Could you check a few things on this drawing? It's one solid part, dimensions in mm from its lowest x, y, z. Round coordinates to 2 decimals unless told otherwise and drop trailing zeros. Write each loop counter-clockwise with the first axis right and the second up, starting at its lowest first coordinate (ties: lowest second). Pieces come first, ordered by that corner, then holes. Notation, with made-up numbers: (20.25, 39) - (51.25, 39) arc R22 cw to (51.25, 72) - close; hole circle Ø9 at (24, -4.5). An arc over 180 degrees is marked (long way). One line per question, with ' | ' between items. Start each with the question number.
(1) Imagine slicing it at B-B (z = 4.25). Write out the boundary of the cut face in (x, y).
(2) Imagine slicing it at C-C (y = 0.5). Write out the boundary of the cut face in (x, z).
(3) Thinking about a two-plate mould opening in Z: for the marked faces 1, 2 and 3, which applies, pulls with the +Z half, pulls with the -Z half, needs draft (parallel to the pull), parting line crosses it, or undercut?
(4) If I drill on L1, parallel to X at y = 0.35, z = 3.65; L2, parallel to X at y = 0.7, z = 2.5; L3, parallel to Z at x = 1.25, y = 0.6, over which ranges is the centre line in solid material (lowest first)?
(5) Imagine slicing it at D-D (x = 0.7). Write out the boundary of the cut face in (y, z).
(6) Will this pin go through, and if not, where does the flat tip stop? pin 1 (1.6 mm diameter, centred on x = 2.4, z = 5, fed in from -Y).
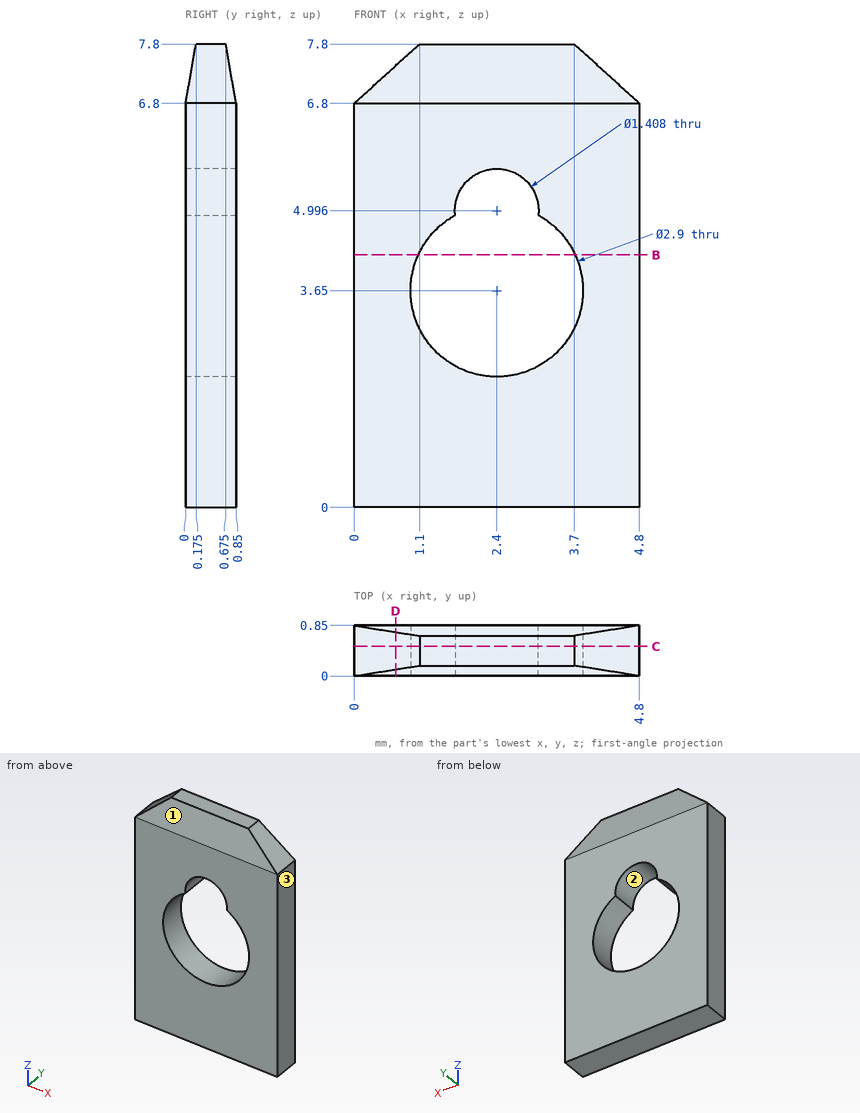
Check sheet entries:
1) outline: (0, 0) - (1.08, 0) - (1.08, 0.85) - (0, 0.85) - close; (3.72, 0) - (4.8, 0) - (4.8, 0.85) - (3.72, 0.85) - close
2) outline: (0, 0) - (4.8, 0) - (4.8, 6.8) - (3.7, 7.8) - (1.1, 7.8) - (0, 6.8) - close; hole (1.7, 4.92) arc R1.45 ccw (long way) to (3.1, 4.92) arc R0.7 ccw (long way) to start
3) face 1: pulls with the +Z half | face 2: undercut | face 3: needs draft
4) L1: 0 to 0.95, 3.85 to 4.8 | L2: 0 to 1.52, 3.28 to 4.8 | L3: 0 to 2.77, 4.53 to 7.8
5) outline: (0, 0) - (0.85, 0) - (0.85, 6.8) - (0.74, 7.44) - (0.11, 7.44) - (0, 6.8) - close
6) pin 1: y = 0
